Geometry check sheet. Reference: the model listing, model coordinates, mm. Face numbers are marked on the shaded views. A direction names the side the tool comes from. Give positions to 0.01 mm unless a question says otherwise; leave off trailing zeros. Write each loop counter-clockwise with the first axis right and the second up, starting at its lowest first coordinate (ties: lowest second). Pieces come first, ordered by that corner, then holes. Notation, with made-up numbers: M -17,78.25 L -1,78.25 A11 ccw -1,87.25 Z; hole C -20.5,24.5 d5. An arc over 180 degrees is marked long. One line per item, written item: value. Start each with the question number.
1. Scan lines: line 1 (Y direction, x = 3, z = 50.5); line 2 (X direction, y = 8, z = 31); line 3 (Z direction, x = 28.5, y = 7.5). Record each from-to range of solid material in increasing order.
2. Cross-section at C-C on y = 14. Record the cut outline in (x, z).
3. Tool access check on the marked faces 4 and 5. Record the directions out of +Z, -Z, +X, -X, +Y, -Y that give a thin tool (end or side, any length) a straight path to the whole face; none if there is none.
4. Release check for a two-part mould opening along X. For the marked faces 1, 2 and 3 record: pulls with the +X half, pulls with the -X half, needs draft (parallel to the pull), parting line crosses it, or undercut.
5. Cross-section at A-A on x = 21. Record the cut outline in (y, z), then the cut area to 3 significant figures.
6. Cross-section at B-B on z = 43.5. Record the cut outline in (x, y), then the cut area to 3 significant figures.
7. Gauge pin test, flat end, axial feed: pin 1 (9 mm diameter, centred on x = 1, y = -4.5, fed in from +Z). Record the tip position at first contact, or that the pin passes through.
8. Cross-section at D-D on z = 3.5. Record the cut outline in (x, y).
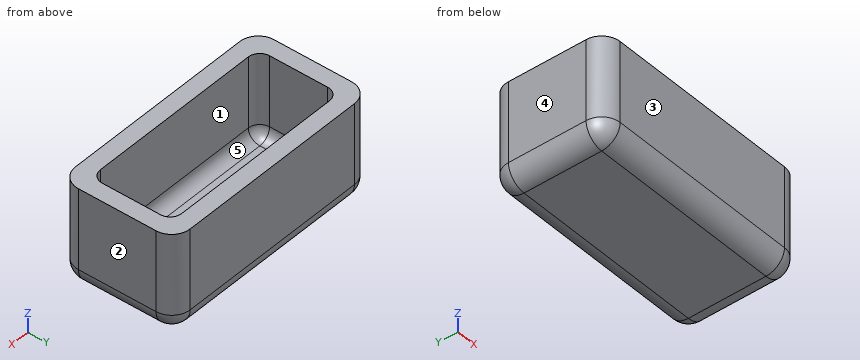
from build123d import *

# Parameters (mm, degrees)
F0_W     = 122.8482164443
F0_H     = 60.7441384345
F1_DEPTH = 52.578
F2_T     = -8.89
F3_R     = 9.8113639175
F4_R     = 6.1321024484


with BuildPart() as f1:
    # F0 (on Top) → F1 (new body)
    with BuildSketch(Plane.XY):
        with Locations((2.0399149507, 0.6799725816)):
            Rectangle(F0_W, F0_H)
    extrude(amount=F1_DEPTH)

    # F2
    f2_openings = [f1.faces().sort_by_distance(p)[0] for p in [
        (2.039915, 0.679973, 52.578),
    ]]
    offset(amount=F2_T, openings=f2_openings)

    # F3
    f3_edges = [f1.edges().sort_by_distance(p)[0] for p in [
        (-59.384193, -29.692097, 26.289),
        (2.039915, -29.692097, 0),
        (2.039915, 31.052042, 0),
        (-59.384193, 0.679973, 0),
        (63.464023, 0.679973, 0),
        (-59.384193, 31.052042, 26.289),
        (63.464023, 31.052042, 26.289),
        (63.464023, -29.692097, 26.289),
    ]]
    fillet(f3_edges, radius=F3_R)

    # F4
    f4_edges = [f1.edges().sort_by_distance(p)[0] for p in [
        (2.039915, 22.162042, 8.89),
        (-50.494193, 0.679973, 8.89),
        (2.039915, -20.802097, 8.89),
        (54.574023, 0.679973, 8.89),
        (-50.494193, -20.802097, 30.734),
        (-50.494193, 22.162042, 30.734),
        (54.574023, -20.802097, 30.734),
        (54.574023, 22.162042, 30.734),
    ]]
    fillet(f4_edges, radius=F4_R)


solid = f1.part
Report:
1. line 1: y = -29.69 to -20.8, 22.16 to 31.05
1. line 2: x = -59.38 to -50.49, 54.57 to 63.46
1. line 3: z = 0 to 8.89
2. outline: M -59.38,9.81 A9.81 ccw -49.57,0 L 53.65,0 A9.81 ccw 63.46,9.81 L 63.46,52.58 L 54.57,52.58 L 54.57,15.02 A6.13 cw 48.44,8.89 L -44.36,8.89 A6.13 cw -50.49,15.02 L -50.49,52.58 L -59.38,52.58 Z
3. face 4: +Z, -Z, -X, +Y, -Y
3. face 5: +Z
4. face 1: undercut
4. face 2: pulls with the +X half
4. face 3: needs draft
5. outline: M -29.69,9.81 A9.81 ccw -19.88,0 L 21.24,0 A9.81 ccw 31.05,9.81 L 31.05,52.58 L 22.16,52.58 L 22.16,15.02 A6.13 cw 16.03,8.89 L -14.67,8.89 A6.13 cw -20.8,15.02 L -20.8,52.58 L -29.69,52.58 Z
5. area: 1,290 mm^2
6. outline: M -59.38,-19.88 A9.81 ccw -49.57,-29.69 L 53.65,-29.69 A9.81 ccw 63.46,-19.88 L 63.46,21.24 A9.81 ccw 53.65,31.05 L -49.57,31.05 A9.81 ccw -59.38,21.24 Z; hole M -50.49,-14.67 A6.13 ccw -44.36,-20.8 L 48.44,-20.8 A6.13 ccw 54.57,-14.67 L 54.57,16.03 A6.13 ccw 48.44,22.16 L -44.36,22.16 A6.13 ccw -50.49,16.03 Z
6. area: 2,900 mm^2
7. pin 1: stops at z = 8.89
8. outline: M -57.08,-19.88 A7.51 ccw -49.57,-27.39 L 53.65,-27.39 A7.51 ccw 61.16,-19.88 L 61.16,21.24 A7.51 ccw 53.65,28.75 L -49.57,28.75 A7.51 ccw -57.08,21.24 Z
